Geometry check sheet. Reference: drawing and pictorial views, mm from the part's lowest x, y, z. A direction names the side the tool comes from. Round coordinates to 2 decimals unless told otherwise and drop trailing zeros. Write each loop counter-clockwise with the first axis right and the second up, starting at its lowest first coordinate (ties: lowest second). Pieces come first, ordered by that corner, then holes. Notation, with made-up numbers: (-15, -34.5) - (-3, -34.5) arc R22 cw to (-3, -11.5) - close; hole circle Ø8 at (52.25, -17.5). An arc over 180 degrees is marked (long way). Use one line per item in the form item = value. Start each with the question number.
1) Section check A-A (z = 27.5). Record the boundary of the cut face in (x, y), then the cut area to 3 significant figures.
2) Scan lines: probe 1 along Y at (x, z) = (49, 11.5); probe 2 along Z at (x, y) = (78.5, 7); probe 3 along X at (y, z) = (39, 13.25). Record each from-to range of solid material in increasing order.
3) Section check B-B (x = 45). Record the boundary of the cut face in (y, z), then the cut area to 3 significant figures.
4) Gauge pin test, flat ends, axial feed: P1, Ø4, axis at x = 66.5, z = 5, coming from the +Y side; P2, Ø4, axis at y = 58, z = 7.5, coming from the -X side; P3, Ø2, axis at y = 38.5, z = 10, coming from the +X side. Record the tip position at first contact, or that the pin passes through.
5) Section check C-C (y = 92). Record the boundary of the cut face in (x, z).
6) Section check D-D (z = 2.25). Record the boundary of the cut face in (x, y).
7) Set-up check for the marked faces 1, 2, 3 and 4: record each of +Z, -Z, +X, -X, +Y, -Y from which the full face is reachable in a straight line by a thin tool's end or side.
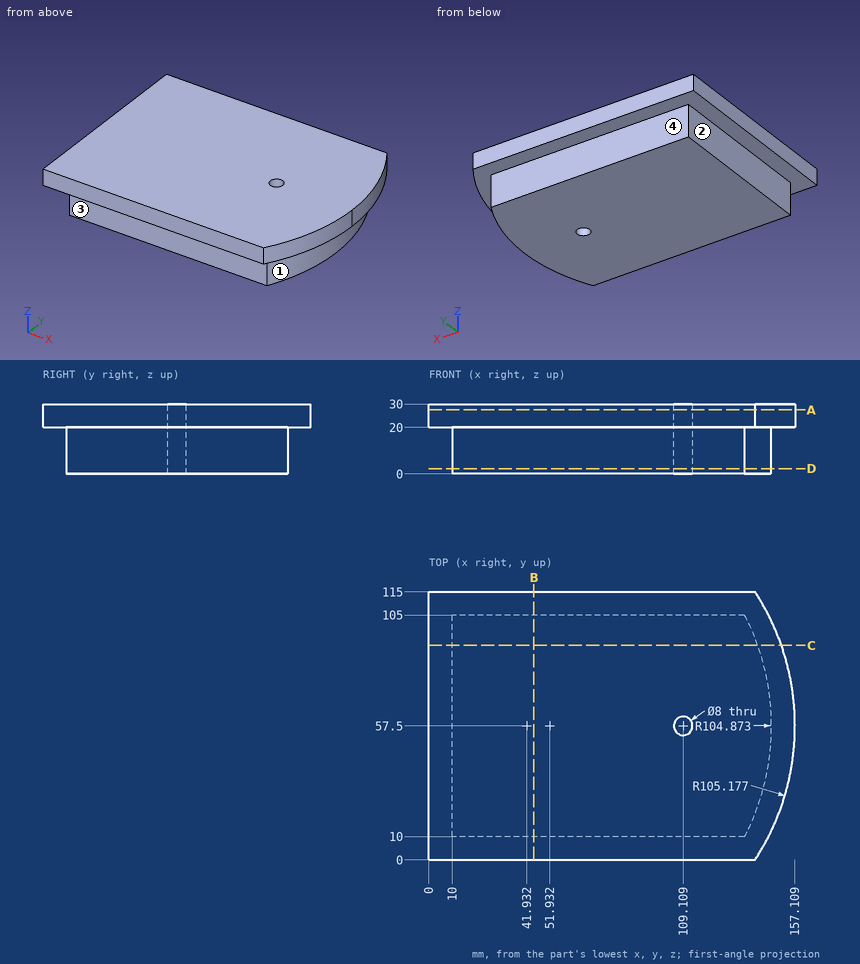
Results are:
q1.outline = (0, 0) - (140, 0) arc R105.18 ccw to (140, 115) - (0, 115) - close; hole circle Ø8 at (109.11, 57.5)
q1.area = 17,400 mm²
q2.probe_1 = 10 to 105
q2.probe_2 = 20 to 30
q2.probe_3 = 10 to 145.16
q3.outline = (0, 20) - (10, 20) - (10, 0) - (105, 0) - (105, 20) - (115, 20) - (115, 30) - (0, 30) - close
q3.area = 3,050 mm²
q4.P1 = 105
q4.P2 = 10
q4.P3 = 145.25
q5.outline = (0, 20) - (10, 20) - (10, 0) - (140.97, 0) - (140.97, 20) - (151.29, 20) - (151.29, 30) - (0, 30) - close
q6.outline = (10, 10) - (135.43, 10) arc R104.87 ccw to (135.43, 105) - (10, 105) - close; hole circle Ø8 at (109.11, 57.5)
q7.face_1 = -Z, +X
q7.face_2 = -Z, -X, +Y, -Y
q7.face_3 = -Z, +X, -X, -Y
q7.face_4 = -Z, +X, -X, +Y
